Job drawing, mm, ordinate dimensions from the low corner. One solid piece. A direction names the side the tool comes from. Give positions to 0.01 mm unless a question says otherwise; leave off trailing zeros. Write each loop counter-clockwise with the first axis right and the second up, starting at its lowest first coordinate (ties: lowest second). Pieces come first, ordered by that corner, then holes. Notation, with made-up numbers: (38, -18.75) -> (92, -18.75) arc R23 cw to (92, -3.75) -> close; hole circle Ø7 at (53, -28.75). An arc over 180 degrees is marked (long way). One line per question, with ' | ' between items. Start each with the question number.
(1) Band-saw the part on C-C, the plane z = 24. Give the cut face in (x, y), and give its area (3 significant figures).
(2) Pull direction Y, two halves, no side cores. Call the marked faces 1, 2 and 3: released by +Y, released by -Y, zero draft, split by the parting line, or undercut.
(3) Drill centre lines: probe 1 along Z at (x, y) = (63, 15); probe 2 along X at (y, z) = (19, 10); probe 3 along X at (y, z) = (3, 26). Where is each one in solid material? Low to high. Write a range as from..to.
(4) Pin check, flat tips, straight feed: P1, Ø14.5, axis at x = 107.95, y = 19.05, coming from the +Z side; P2, Ø5, axis at x = 66.5, y = 4.5, coming from the +Z side; P3, Ø3, axis at x = 89.5, y = 11, coming from the +Z side; P4, Ø15, axis at x = 63.5, z = 25.4, coming from the -Y side. Stop position of each tip, or through.
(5) Band-saw the part on B-B, the plane x = 63.5. Give the cut face in (y, z), and give its area (3 significant figures).
(6) Tool access for the marked faces 4, 5 and 6: list every direction of +Z, -Z, +X, -X, +Y, -Y with a clear straight run to the whole face (end or side of a thin tool).
(7) Band-saw the part on A-A, the plane y = 19.05. Give the cut face in (x, z).
(8) Band-saw the part on D-D, the plane z = 7.5. Give the cut face in (x, y).
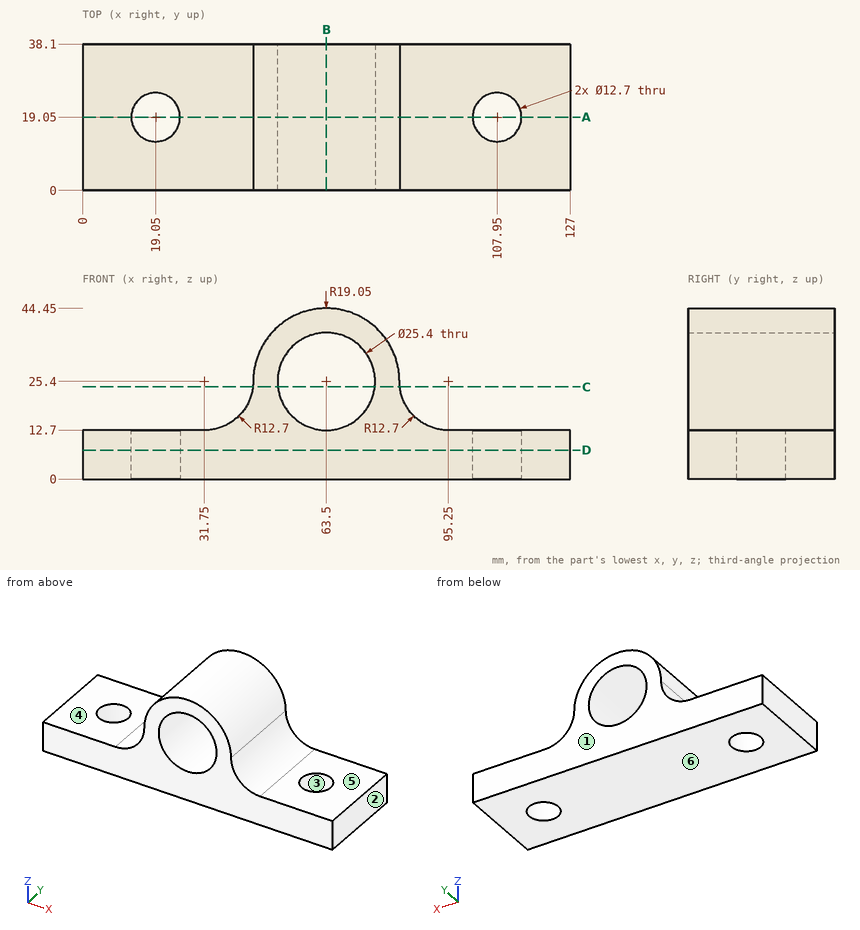
Results:
1) outline: (44.37, 0) -> (50.88, 0) -> (50.88, 38.1) -> (44.37, 38.1) -> close; (76.12, 0) -> (82.63, 0) -> (82.63, 38.1) -> (76.12, 38.1) -> close | area: 496 mm²
2) face 1: released by +Y | face 2: zero draft | face 3: undercut
3) probe 1: z = 0..12.71, 38.09..44.44 | probe 2: x = 0..12.7, 25.4..101.6, 114.3..127 | probe 3: x = 44.46..50.81, 76.19..82.54
4) P1: stops at z = 12.7 | P2: stops at z = 44.44 | P3: stops at z = 14.97 | P4: passes through
5) outline: (0, 0) -> (38.1, 0) -> (38.1, 12.7) -> (0, 12.7) -> close; (0, 38.1) -> (38.1, 38.1) -> (38.1, 44.45) -> (0, 44.45) -> close | area: 726 mm²
6) face 4: +Z, -X, +Y, -Y | face 5: +Z, +X, +Y, -Y | face 6: -Z, +X, -X, +Y, -Y
7) outline: (0, 0) -> (12.7, 0) -> (12.7, 12.7) -> (0, 12.7) -> close; (25.4, 0) -> (101.6, 0) -> (101.6, 12.7) -> (95.25, 12.7) arc R12.7 cw to (82.55, 25.4) arc R19.05 ccw to (44.45, 25.4) arc R12.7 cw to (31.75, 12.7) -> (25.4, 12.7) -> close; (114.3, 0) -> (127, 0) -> (127, 12.7) -> (114.3, 12.7) -> close; hole circle Ø25.4 at (63.5, 25.4)
8) outline: (0, 0) -> (127, 0) -> (127, 38.1) -> (0, 38.1) -> close; hole circle Ø12.7 at (19.05, 19.05); hole circle Ø12.7 at (107.95, 19.05)
